The figure shows three views and two pictorial views of one solid part (mm, origin at its lowest corner). Answer the questions. Give positions to 0.01 mm unless a question says otherwise; leave off trailing zeros. Write each loop counter-clockwise with the first axis right and the second up, starting at its lowest first coordinate (ties: lowest second). Pieces come first, ordered by that corner, then holes. Notation, with made-up numbers: (-24, 43.25) -> (7, 43.25) arc R16 cw to (7, 58.25) -> close; hole circle Ø7 at (5, 52). An arc over 180 degrees is marked (long way). Use a Markdown table: item, result.
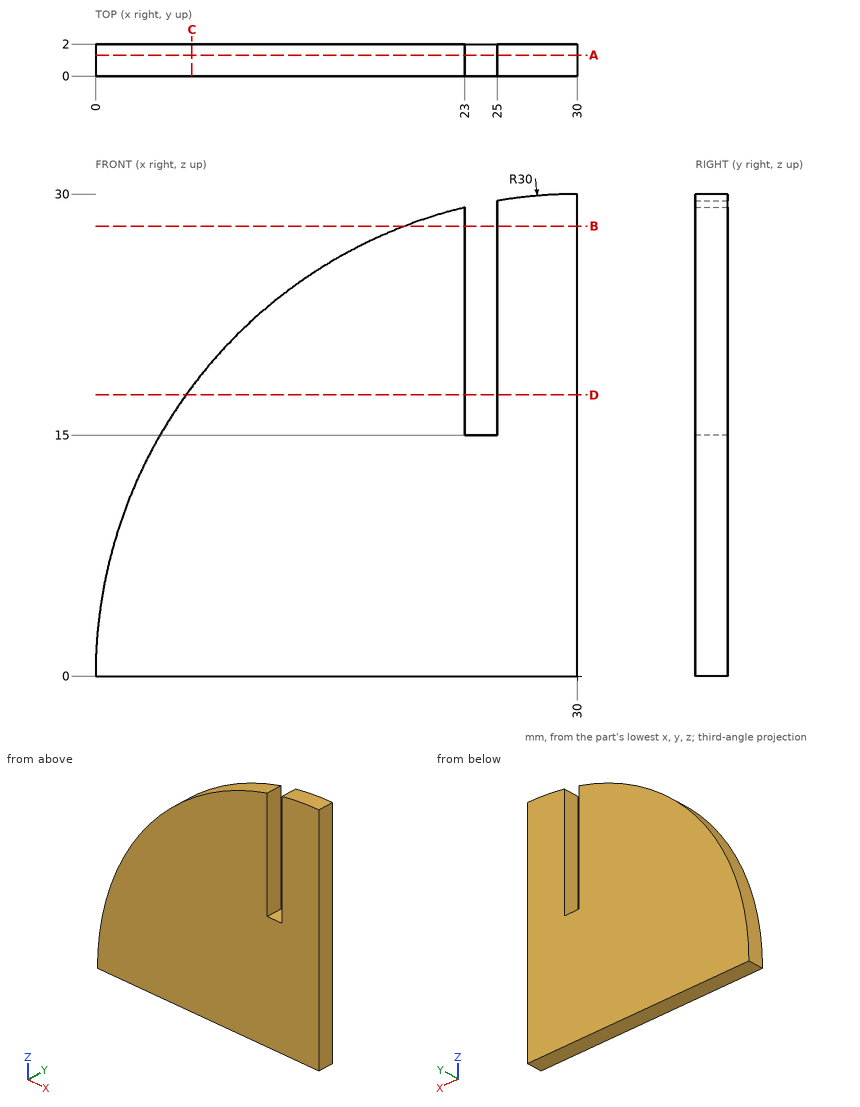
Item 1: A cutting plane is placed at C-C (x = 6). Give the vertices of the cut face in (y, z), then the cut area to 3 significant figures.
Return value:
| item | result |
|---|---|
| outline | (0, 0) -> (2, 0) -> (2, 18) -> (0, 18) -> close |
| area | 36.0 mm^2 |
Item 2: Straight lines are drawn through the part: line 1 along Z through (x, y) = (24, 1.55); line 2 along X through (y, z) = (1.3, 17.75); line 3 along X through (y, z) = (0.5, 16.5). For each, find the intervals that lie inside material, in ascending order. Write a range as [from, to].
Return value:
| item | result |
|---|---|
| line 1 | [0, 15] |
| line 2 | [5.81, 23], [25, 30] |
| line 3 | [4.95, 23], [25, 30] |
Item 3: This flat-tipped pin is pushed along its axis until it touches: P1, Ø1, axis at y = 0.5, z = 20, coming from the -X side. Where does it stop, or does it pass through?
Return value:
| item | result |
|---|---|
| P1 | x = 7.2 |
Item 4: A cutting plane is placed at A-A (y = 1.3). Give the vertices of the cut face in (x, z), then the cut area to 3 significant figures.
Return value:
| item | result |
|---|---|
| outline | (0, 0) -> (30, 0) -> (30, 30) arc R30 ccw to (25, 29.58) -> (25, 15) -> (23, 15) -> (23, 29.17) arc R30 ccw to start |
| area | 678 mm^2 |
Item 5: A cutting plane is placed at D-D (z = 17.5). Give the vertices of the cut face in (x, y), then the cut area to 3 significant figures.
Return value:
| item | result |
|---|---|
| outline | (5.63, 0) -> (23, 0) -> (23, 2) -> (5.63, 2) -> close; (25, 0) -> (30, 0) -> (30, 2) -> (25, 2) -> close |
| area | 44.7 mm^2 |
Item 6: A cutting plane is placed at B-B (z = 28). Give the vertices of the cut face in (x, y).
Return value:
| item | result |
|---|---|
| outline | (19.23, 0) -> (23, 0) -> (23, 2) -> (19.23, 2) -> close; (25, 0) -> (30, 0) -> (30, 2) -> (25, 2) -> close |
